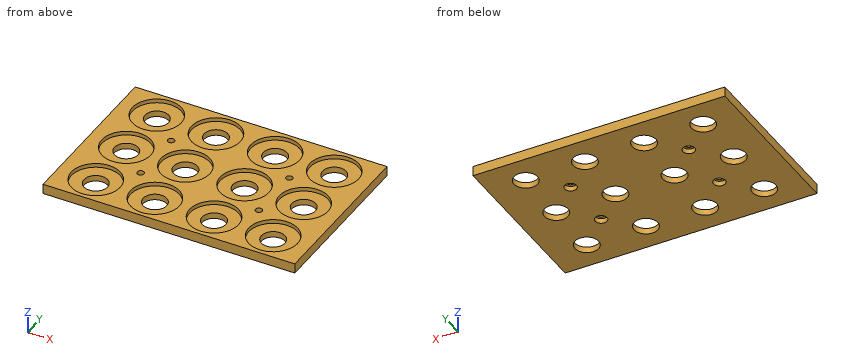
Autodesk Fusion 360 part; units mm, degrees
sketch "Sketch1" plane through (0, 0, 0) normal (0, 0, 1) x (1, 0, 0)
  line L0 (0, 0) -> (127.76, 0)
  line L1 (127.76, 0) -> (127.76, -85.48)
  line L2 (127.76, -85.48) -> (0, -85.48)
  line L3 (0, -85.48) -> (0, 0)
  dimension "d1" = 127.76
  dimension "d2" = 85.48
extrude "Extrude1" add sketch "Sketch1" along normal blind 5
sketch "Sketch7" plane through (0, 0, 5) normal (0, 0, 1) x (-1, 0, 0)
  line L0 (0, 85.48) -> (-127.76, 85.48)
  line L1 (-127.76, 85.48) -> (-127.76, 0)
  line L2 (-127.76, 0) -> (0, 0)
  line L3 (0, 0) -> (0, 85.48)
  point P0 (-18.875, 14.4325)
  point P1 (-48.878, 14.4325)
  point P2 (-78.881, 14.4325)
  point P3 (-108.884, 14.4325)
  point P4 (-18.875, 42.74)
  point P5 (-48.878, 42.74)
  point P6 (-78.881, 42.74)
  point P7 (-108.884, 42.74)
  point P8 (-18.875, 71.0475)
  point P9 (-48.878, 71.0475)
  point P10 (-78.881, 71.0475)
  point P11 (-108.884, 71.0475)
  dimension "d42" = -30.003
  dimension "d43" = 28.3075
hole "Hole1" at (18.875, -14.4325, 5) at (18.875, -42.74, 5) at (18.875, -71.0475, 5) at (48.878, -71.0475, 5) at (48.878, -42.74, 5) at (48.878, -14.4325, 5) at (78.881, -14.4325, 5) at (78.881, -42.74, 5) at (78.881, -71.0475, 5) at (108.884, -71.0475, 5) at (108.884, -42.74, 5) at (108.884, -14.4325, 5) direction (0, 0, -1) diameter 12 depth 13 tip angle 180 counterbore diameter 24.8 counterbore depth 2
sketch "Sketch8" plane through (0, 0, 0) normal (0, 0, -1) x (1, 0, 0)
  circle A0 centre (108.884, 42.74) radius 6
  circle A1 centre (78.881, 71.0475) radius 6
  circle A2 centre (78.881, 14.4325) radius 6
  circle A3 centre (48.878, 42.74) radius 6
  circle A4 centre (18.875, 71.0475) radius 6
  circle A5 centre (18.875, 14.4325) radius 6
  circle A6 centre (18.875, 42.74) radius 6
  circle A7 centre (48.878, 71.0475) radius 6
  circle A8 centre (48.878, 14.4325) radius 6
  circle A9 centre (78.881, 42.74) radius 6
  circle A10 centre (108.884, 71.0475) radius 6
  circle A11 centre (108.884, 14.4325) radius 6
  line L0 (127.76, 85.48) -> (0, 85.48)
  line L1 (0, 85.48) -> (0, 0)
  line L2 (0, 0) -> (127.76, 0)
  line L3 (127.76, 0) -> (127.76, 85.48)
  point P0 (33.877, 28.587)
  point P1 (93.883, 28.587)
  point P2 (33.877, 56.8945)
  point P3 (93.883, 56.8945)
  dimension "d52" = 60.006
  dimension "d53" = 28.3075
hole "Hole3" at (33.877, -56.8945, 0) at (33.877, -28.587, 0) at (93.883, -56.8945, 0) at (93.883, -28.587, 0) direction (0, 0, 1) diameter 3.4 depth 20 tip angle 118 counterbore diameter 6 counterbore depth 2.5
Work out the finished part from the listing and answer in its coordinate system (mm). Round coordinates to 2 decimals unless told otherwise and drop trailing zeros. Write each loop counter-clockwise with the first axis right and the second up, starting at its lowest first coordinate (ties: lowest second). Pieces come first, ordered by that corner, then holes. Notation, with made-up numbers: (49, 56.25) -> (88, 56.25) arc R18 cw to (88, 74.25) -> close; hole circle Ø3 at (7.5, 75). An arc over 180 degrees is marked (long way). Answer as CSV lines item,"result". Start each with the question number.
(1) The part is cut by section D-D, the plane y = -6. Give the vertices of the cut face in (x, z), then the cut area to 3 significant figures.
(2) Each of these flat-tipped pins is pushed along its axis until it touches: pin 1 (12.5 mm diameter, centred on x = 53, y = -15, fed in from +Z); pin 2 (11 mm diameter, centred on x = 108.884, y = -42.74, fed in from -Z). Where does it stop, or does it pass through?
(3) The part is cut by section A-A, the plane z = 3.8. Give the number of separate pieces and of enclosed holes in the cut face, then the cut area to 3 significant figures.
(4) The part is cut by section C-C, the plane x = 118. Give the vertices of the cut face in (y, z), then the cut area to 3 significant figures.
(5) Find the intervals of material crossed by probe 1 along X at (y, z) = (-15, 4.6) (3 decimals); probe 2 along Y at (x, z) = (79, 2.3); probe 3 along X at (y, z) = (-9, 2.05), in increasing order.
Output values:
1,outline,"(0, 0) -> (127.76, 0) -> (127.76, 5) -> (117.98, 5) -> (117.98, 3) -> (99.79, 3) -> (99.79, 5) -> (87.97, 5) -> (87.97, 3) -> (69.79, 3) -> (69.79, 5) -> (57.97, 5) -> (57.97, 3) -> (39.79, 3) -> (39.79, 5) -> (27.97, 5) -> (27.97, 3) -> (9.78, 3) -> (9.78, 5) -> (0, 5) -> close"
1,area,"493 mm²"
2,pin 1,"stops at z = 3"
2,pin 2,"passes through"
3,separate pieces,"1"
3,enclosed holes,"16"
3,area,"5,090 mm²"
4,outline,"(-85.48, 0) -> (0, 0) -> (0, 5) -> (-6.03, 5) -> (-6.03, 3) -> (-22.84, 3) -> (-22.84, 5) -> (-34.33, 5) -> (-34.33, 3) -> (-51.15, 3) -> (-51.15, 5) -> (-62.64, 5) -> (-62.64, 3) -> (-79.45, 3) -> (-79.45, 5) -> (-85.48, 5) -> close"
4,area,"327 mm²"
5,probe 1,"x = 0 to 6.488, 31.262 to 36.491, 61.265 to 66.494, 91.268 to 96.497, 121.271 to 127.76"
5,probe 2,"y = -85.48 to -77.05, -65.05 to -48.74, -36.74 to -20.43, -8.43 to 0"
5,probe 3,"x = 0 to 16.33, 21.42 to 46.33, 51.43 to 76.33, 81.43 to 106.34, 111.43 to 127.76"
